Work out the finished part from the listing and answer in its coordinate system (mm). Face numbers are marked on the shaded views. A direction names the side the tool comes from. Round coordinates to 2 decimals unless told otherwise and drop trailing zeros. Loops run counter-clockwise (first coordinate to the right, second up) from the corner with the lowest first, then second, coordinate; pieces in that order, holes last. Notation, with made-up numbers: M 1.5,-13 L 24.5,-13 A24 ccw 24.5,6 Z; hole C -18.5,39.5 d7. An arc over 180 degrees is marked long. One line per item, written item: value.
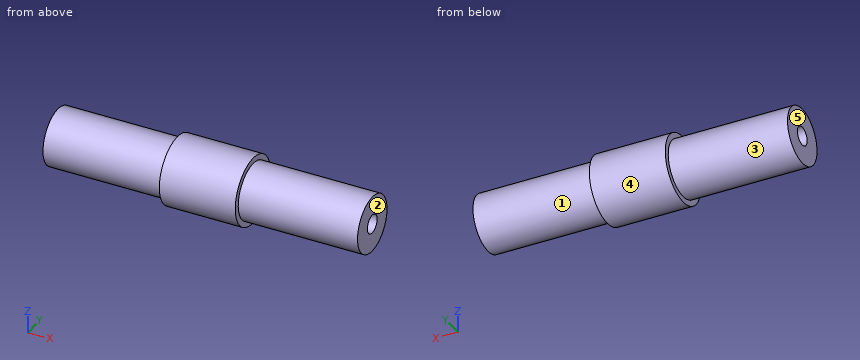
```python
from build123d import *

# Parameters (mm, degrees)
SKETCH_1_R          = 6
EXTRUDE_1_DEPTH     = 13.4
SKETCH_2_R          = 5
EXTRUDE_2_DEPTH     = 21.05
EXTRUDE_START       = 21.05
SKETCH_3_R          = 5
EXTRUDE_3_DEPTH     = 21.05
SKETCH_4_R          = 1.65
CUT_EXTRUDE_1_DEPTH = 10
CUT_EXTRUDE_START   = -10
SKETCH_5_R          = 1.65
CUT_EXTRUDE_2_DEPTH = 10


with BuildPart() as part:
    # ｽｹｯﾁ1 → ﾎﾞｽ - 押し出し1 (new body)
    with BuildSketch(Plane(origin=(0, 0, 0), x_dir=(0, 0, -1), z_dir=(1, 0, 0))):
        Circle(SKETCH_1_R)
    extrude(amount=EXTRUDE_1_DEPTH)

    # ｽｹｯﾁ2 → ﾎﾞｽ - 押し出し2 (add)
    with BuildSketch(Plane(origin=(13.4, 0, 0), x_dir=(0, 0, -1), z_dir=(1, 0, 0))):
        Circle(SKETCH_2_R)
    extrude(amount=EXTRUDE_2_DEPTH)

    # ｽｹｯﾁ3 → ﾎﾞｽ - 押し出し3 (add)
    with BuildSketch(Plane.ZY.offset(EXTRUDE_START)):
        with Locations(Location((0, 0, 0), (0, 0, 180))):
            Circle(SKETCH_3_R)
    extrude(amount=-EXTRUDE_3_DEPTH)

    # ｽｹｯﾁ4 → ｶｯﾄ - 押し出し1 (cut)
    with BuildSketch(Plane(origin=(34.45, 0, 0), x_dir=(0, 0, -1), z_dir=(1, 0, 0))):
        Circle(SKETCH_4_R)
    extrude(amount=-CUT_EXTRUDE_1_DEPTH, mode=Mode.SUBTRACT)

    # ｽｹｯﾁ5 → ｶｯﾄ - 押し出し2 (cut)
    with BuildSketch(Plane.ZY.offset(21.05).offset(CUT_EXTRUDE_START)):
        with Locations(Location((0, 0, 0), (0, 0, 180))):
            Circle(SKETCH_5_R)
    extrude(amount=CUT_EXTRUDE_2_DEPTH, mode=Mode.SUBTRACT)


solid = part.part
```
1) Find section A-A (z = 0). Give the vertices of the cut face in (x, y).
Check values:
outline: M -21.05,-5 L 0,-5 L 0,-6 L 13.4,-6 L 13.4,-5 L 34.45,-5 L 34.45,-1.65 L 24.45,-1.65 L 24.45,1.65 L 34.45,1.65 L 34.45,5 L 13.4,5 L 13.4,6 L 0,6 L 0,5 L -21.05,5 L -21.05,1.65 L -11.05,1.65 L -11.05,-1.65 L -21.05,-1.65 Z
2) Each of these flat-tipped pins is pushed along its axis until it touches: pin 1 (3 mm diameter, centred on x = -9, y = 2.5, fed in from -Z); pin 2 (6 mm diameter, centred on x = 16, y = -4, fed in from +Z); pin 3 (2 mm diameter, centred on x = 4, z = -0.5, fed in from -Y); pin 4 (1.5 mm diameter, centred on x = 1.5, y = 4.5, fed in from -Z). Where does it stop, or does it pass through?
Check values:
pin 1: z = -4.9
pin 2: z = 5.45
pin 3: y = -6
pin 4: z = -4.68
3) Find section C-C (x = 26). Give the vertices of the cut face in (y, z).
Check values:
outline: C 0,0 d10; hole C 0,0 d3.3
4) Find the intervals of material crossed by probe 1 along Y at (x, z) = (-15, 0); probe 2 along X at (y, z) = (5, 2.5); probe 3 along Z at (x, y) = (10.5, -0.25), in increasing order. Write a range as from..to.
Check values:
probe 1: -5..-1.65, 1.65..5
probe 2: 0..13.4
probe 3: -5.99..5.99
5) Find section D-D (x = 8). Give the vertices of the cut face in (y, z).
Check values:
outline: C 0,0 d12
6) The mould has two halves that part along Y. Classify the marked faces 4 and 5: +Y half, -Y half, draft (parallel to the pull), parting line (faces both ways), or undercut.
Check values:
face 4: parting line
face 5: draft
7) Find section B-B (y = 0.75). Give the vertices of the cut face in (x, z).
Check values:
outline: M -21.05,-4.94 L 0,-4.94 L 0,-5.95 L 13.4,-5.95 L 13.4,-4.94 L 34.45,-4.94 L 34.45,-1.47 L 24.45,-1.47 L 24.45,1.47 L 34.45,1.47 L 34.45,4.94 L 13.4,4.94 L 13.4,5.95 L 0,5.95 L 0,4.94 L -21.05,4.94 L -21.05,1.47 L -11.05,1.47 L -11.05,-1.47 L -21.05,-1.47 Z
8) For the marked faces 1, 2 and 3, determine the directions among +Z, -Z, +X, -X, +Y, -Y from which every point of the face is accessible in a straight line to the end or side of a thin tool.
Check values:
face 1: +X
face 2: +Z, -Z, +X, +Y, -Y
face 3: -X
